The model under review builds one solid part; all positions refer to its coordinate system, in mm. Coordinates: 2 decimals unless noted, no trailing zeros. Order: outer loops, then holes, each group sorted by start corner. A loop starts at its lowest first (then second) coordinate and runs counter-clockwise, first axis right, second up. Notation, with made-up numbers: M -26,52 L 7,52 A25 ccw 7,82 Z; hole C 86,75 d3. An arc over 180 degrees is marked long. Answer in a Markdown table with one row per item.
from build123d import *

# Parameters (mm, degrees)
F1_DEPTH = 25
F2_DEPTH = 89
F4_D     = 5
F5_DEPTH = 25


with BuildPart() as f1:
    # F0 (on Top) → F1 (new body)
    with BuildSketch(Plane.XY):
        with BuildLine():
            ThreePointArc((-64.6422651169, 61.7318101091), (-104.509721445, 40.0797605591), (-75.6510277108, 5.0740307461))
            Line((-75.6510277108, 5.0740307461), (-75.6510277108, 20.4725478984))
            ThreePointArc((-75.6510277108, 20.4725478984), (-85.5504441422, 44.3718533068), (-61.6511387339, 34.4724368753))
            Line((-61.6511387339, 34.4724368753), (-46.2526215815, 34.4724368753))
            ThreePointArc((-46.2526215815, 34.4724368753), (-51.279873074, 50.91363831), (-64.6422651169, 61.7318101091))
        make_face()
        with BuildLine():
            Line((-46.2526215815, 34.4724368753), (75.6510277108, 34.4724368753))
            ThreePointArc((75.6510277108, 34.4724368753), (4.192505753, 41.3504150705), (-64.6422651169, 61.7318101091))
            ThreePointArc((-64.6422651169, 61.7318101091), (-51.279873074, 50.91363831), (-46.2526215815, 34.4724368753))
        make_face()
        with BuildLine():
            Line((-75.6510277108, 20.4725478984), (-75.6510277108, 5.0740307461))
            ThreePointArc((-75.6510277108, 5.0740307461), (-54.8632153807, 13.6846245453), (-46.2526215815, 34.4724368753))
            Line((-46.2526215815, 34.4724368753), (-61.6511387339, 34.4724368753))
            ThreePointArc((-61.6511387339, 34.4724368753), (-65.7516112793, 24.5730204439), (-75.6510277108, 20.4725478984))
        make_face()
        with BuildLine():
            Line((-75.6510277108, -34.4724368753), (75.6510277108, -34.4724368753))
            Line((75.6510277108, -34.4724368753), (75.6510277108, 34.4724368753))
            Line((75.6510277108, 34.4724368753), (-46.2526215815, 34.4724368753))
            ThreePointArc((-46.2526215815, 34.4724368753), (-54.8632153807, 13.6846245453), (-75.6510277108, 5.0740307461))
            Line((-75.6510277108, 5.0740307461), (-75.6510277108, -34.4724368753))
        make_face()
    extrude(amount=F1_DEPTH)

    # F0 (on Top) → F2 (join, symmetric)
    with BuildSketch(Plane.XY):
        with BuildLine():
            ThreePointArc((-61.6511387339, 34.4724368753), (-85.5504441422, 44.3718533068), (-75.6510277108, 20.4725478984))
            Line((-75.6510277108, 20.4725478984), (-75.6510277108, 34.4724368753))
            Line((-75.6510277108, 34.4724368753), (-61.6511387339, 34.4724368753))
        make_face()
        with BuildLine():
            Line((-75.6510277108, 34.4724368753), (-75.6510277108, 20.4725478984))
            ThreePointArc((-75.6510277108, 20.4725478984), (-65.7516112793, 24.5730204439), (-61.6511387339, 34.4724368753))
            Line((-61.6511387339, 34.4724368753), (-75.6510277108, 34.4724368753))
        make_face()
    extrude(amount=F2_DEPTH, both=True)

    # F4 (through all)
    with Locations(Plane.XY.offset(25)):
        with Locations((-78.5690456042, 54.7676971151), (-67.133374486, 53.123495831), (-58.4019980838, 45.5577151106), (-55.1470667124, 34.4724368753), (-58.4019980838, 23.3871586401), (-67.133374486, 15.8213779197), (-78.5690456042, 14.1771766356), (-89.078266659, 18.9765770782), (-95.32443422, 28.6958035179), (-95.32443422, 40.2490702328), (-89.078266659, 49.9682966725)):
            Hole(F4_D / 2)

    # F5 (add): a face of the model
    f5_faces = [f1.faces().sort_by_distance(p)[0] for p in [
        (-9.2870203621, 6.9469719562, 25),
    ]]
    extrude(f5_faces, amount=F5_DEPTH)


solid = f1.part
(1) Take a section at D-D (x = 45). Write out the cut boundary in (y, z), then the cut area to 3 significant figures.
Report:
| item | result |
|---|---|
| outline | M -34.47,0 L 35.73,0 L 35.73,50 L -34.47,50 Z |
| area | 3,510 mm^2 |
(2) The part is to be moulded in two halves that separate along Y. For faces 1 (the flat face through (-75.651, -14, 25)), 2 (the cylindrical face through (5.18, 41.16, 24.65)), 3 (the cylindrical face through (-80.954, 14.928, 24.65)), say which applies: +Y half, -Y half, draft (parallel to the pull), parting line (faces both ways), or undercut.
Report:
| item | result |
|---|---|
| face 1 | draft |
| face 2 | +Y half |
| face 3 | undercut |
(3) Insertion check: P1, Ø8, axis at x = -78.57, y = 54.77, coming from the -Z side; P2, Ø6, axis at x = -2.5, y = 23, coming from the +Z side; P3, Ø2, axis at x = -87, z = 26, coming from the -Y side. Each pin has a flat end and moves straight along its axis. Give the tip position at first contact, or say it passes through.
Report:
| item | result |
|---|---|
| P1 | z = 0 |
| P2 | z = 50 |
| P3 | y = 6.96 |
(4) To check wall thickness, follow line 1 (Y direction, x = -66, z = 18); line 2 (Z direction, x = 67, y = 3); line 3 (Y direction, x = -78.5, z = 44). State the ranges of each line that lie inside material, in increasing order. Write a range as [from, to].
Report:
| item | result |
|---|---|
| line 1 | [-34.47, 13.59], [18.05, 50.9], [55.35, 62.24] |
| line 2 | [0, 50] |
| line 3 | [5.21, 11.68], [16.68, 52.27], [57.27, 63.73] |
(5) Take a section at B-B (z = 77). Write out the cut boundary in (x, y), then the cut area to 3 significant figures.
Report:
| item | result |
|---|---|
| outline | C -75.65,34.47 d28 |
| area | 616 mm^2 |
(6) Take a section at C-C (y = -9). Write out the cut boundary in (x, z), then the cut area to 3 significant figures.
Report:
| item | result |
|---|---|
| outline | M -75.65,0 L 75.65,0 L 75.65,50 L -75.65,50 Z |
| area | 7,570 mm^2 |
(7) Take a section at A-A (z = 24.5). State how many separate pieces and enclosed holes the cut face has, then the cut area to 3 significant figures.
Report:
| item | result |
|---|---|
| separate pieces | 1 |
| enclosed holes | 11 |
| area | 13,100 mm^2 |
